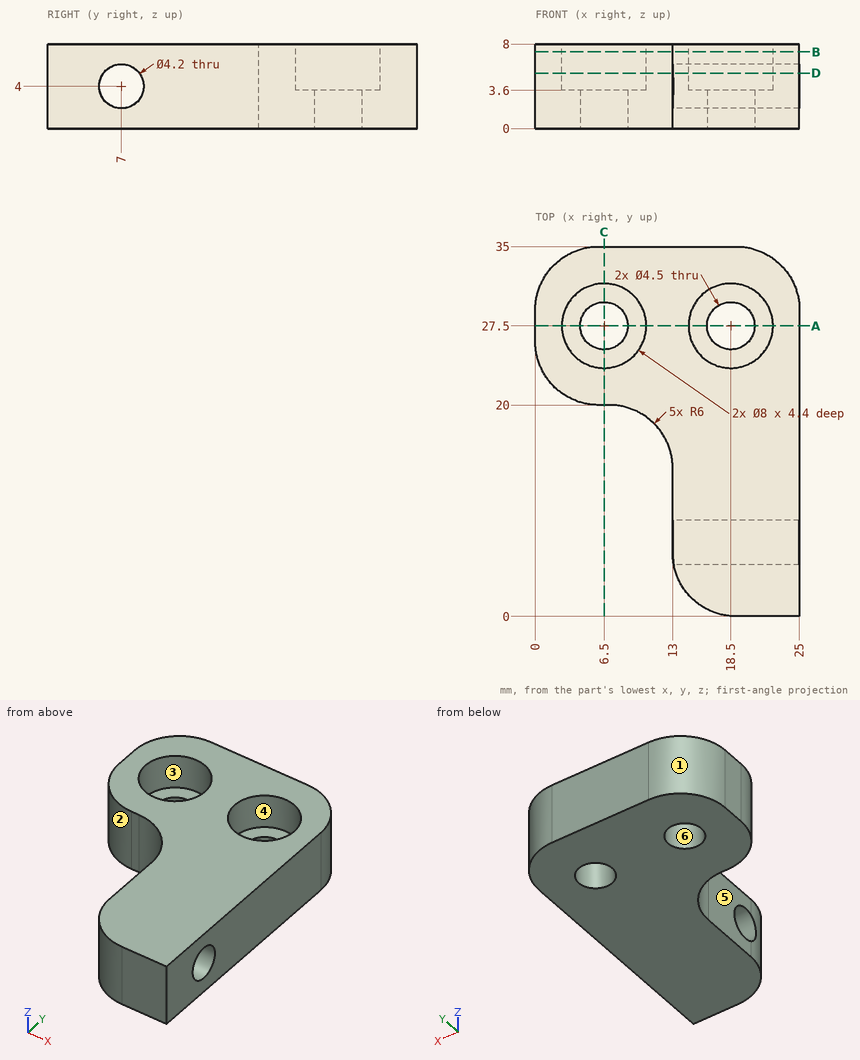
For this review, use the dimensioned drawing (mm, ordinates from the lowest corner) and the shaded views. A direction names the side the tool comes from. Give positions to 0.01 mm unless a question says otherwise; leave off trailing zeros. Order: outer loops, then holes, each group sorted by start corner. A loop starts at its lowest first (then second) coordinate and runs counter-clockwise, first axis right, second up. Notation, with made-up numbers: M 30,54.25 L 76,54.25 A22 cw 76,61.25 Z; hole C -16,-22.75 d8. An arc over 180 degrees is marked long. One line per question, with ' | ' between items. Start each with the question number.
1) Consider section D-D, the plane z = 5.25. Give the boundary of the cut face in (x, y).
2) Clearance check with flat-ended pins moving along their axes: P1, Ø2.5, axis at x = 6.5, y = 27.5, coming from the +Z side (1 decimal); P2, Ø13, axis at x = 18.5, y = 27.5, coming from the -Z side; P3, Ø0.8, axis at x = 6.5, z = 2.5, coming from the -Y side; P4, Ø2.5, axis at x = 19.5, y = 26, coming from the +Z side. State where each tip first meets the part, or that it passes through.
3) Consider section A-A, the plane y = 27.5. Give the boundary of the cut face in (x, z).
4) Consider section C-C, the plane x = 6.5. Give the boundary of the cut face in (y, z).
5) Wall thickness on L1, parallel to Y at x = 17.25, z = 4.75; L2, parallel to Y at x = 18.5, z = 4.55; L3, parallel to Y at x = 6.5, z = 1.35: over which ranges is each line inside the solid? List them lowest first. Write a range as from..to.
6) Mouldability with a two-part tool opening along Y and no side actions: class the marked faces 1, 2 and 3 as pulls with the +Y half, pulls with the -Y half, needs draft (parallel to the pull), parting line crosses it, or undercut.
7) Consider section B-B, the plane z = 7.25. Give the boundary of the cut face in (x, y), then the cut area to 3 significant figures.
8) For the marked faces 4, 5 and 6, list the 3-axis set-ups (+Z, -Z, +X, -X, +Y, -Y) from which the entire face can be reached by the end or side of a thin tool; tool diameter is ignored.
Found:
1) outline: M 0,26 A6 ccw 6,20 L 7,20 A6 cw 13,14 L 13,8.69 L 25,8.69 L 25,29 A6 ccw 19,35 L 6,35 A6 ccw 0,29 Z; M 13.04,5.31 A6 ccw 19,0 L 25,0 L 25,5.31 Z; hole C 6.5,27.5 d8; hole C 18.5,27.5 d8
2) P1: passes through | P2: stops at z = 0 | P3: stops at y = 20 | P4: stops at z = 3.6
3) outline: M 0,0 L 4.25,0 L 4.25,3.6 L 2.5,3.6 L 2.5,8 L 0,8 Z; M 8.75,0 L 16.25,0 L 16.25,3.6 L 14.5,3.6 L 14.5,8 L 10.5,8 L 10.5,3.6 L 8.75,3.6 Z; M 20.75,0 L 25,0 L 25,8 L 22.5,8 L 22.5,3.6 L 20.75,3.6 Z
4) outline: M 20,0 L 25.25,0 L 25.25,3.6 L 23.5,3.6 L 23.5,8 L 20,8 Z; M 29.75,0 L 35,0 L 35,8 L 31.5,8 L 31.5,3.6 L 29.75,3.6 Z
5) L1: y = 0.26..5.04, 8.96..23.7, 31.3..35 | L2: y = 0.02..4.97, 9.03..23.5, 31.5..35 | L3: y = 20..25.25, 29.75..35
6) face 1: pulls with the +Y half | face 2: pulls with the -Y half | face 3: undercut
7) outline: M 0,26 A6 ccw 6,20 L 7,20 A6 cw 13,14 L 13,6 A6 ccw 19,0 L 25,0 L 25,29 A6 ccw 19,35 L 6,35 A6 ccw 0,29 Z; hole C 6.5,27.5 d8; hole C 18.5,27.5 d8 | area: 491 mm²
8) face 4: +Z | face 5: +Z, -Z, -X, -Y | face 6: +Z, -Z
